The listing builds one solid part. Answer for the finished solid, in the listing's coordinates (mm). A direction names the side the tool comes from. Give positions to 0.01 mm unless a question says otherwise; leave off trailing zeros. Write each loop counter-clockwise with the first axis right and the second up, starting at its lowest first coordinate (ties: lowest second). Pieces come first, ordered by that corner, then holes. Notation, with made-up numbers: (64.5, 57) - (69.5, 57) arc R19 ccw to (69.5, 69) - close; hole circle Ø9 at (84, 55.5). An arc over 180 degrees is marked (long way). Return JSON: item names as keys, results as strings.
from build123d import *

# Parameters (mm, degrees)
F1_DEPTH = 10
F2_R     = 10
F3_T     = -1


with BuildPart() as f1:
    # F0 (on Top) → F1 (new body)
    with BuildSketch(Plane.XY):
        Polygon((35.284058, 50.538993), (-54.715942, 50.538993), (-54.715942, -39.461007), (-24.715942, -39.461007), (-24.715942, 20.538993), (5.284058, 20.538993), (5.284058, -39.461007), (35.284058, -39.461007), align=None)
    extrude(amount=F1_DEPTH)

    # F2
    f2_edges = [f1.edges().sort_by_distance(p)[0] for p in [
        (35.284058, 50.538993, 5),
        (35.284058, -39.461007, 5),
        (-24.715942, 20.538993, 5),
        (-24.715942, -39.461007, 5),
        (-54.715942, -39.461007, 5),
        (5.284058, -39.461007, 5),
        (5.284058, 20.538993, 5),
        (-54.715942, 50.538993, 5),
    ]]
    fillet(f2_edges, radius=F2_R)

    # F3
    f3_openings = [f1.faces().sort_by_distance(p)[0] for p in [
        (-9.715942, 49.2662, 10),
    ]]
    offset(amount=F3_T, openings=f3_openings)


solid = f1.part
Item 1: For faces 1 (the face through (20, -38.461, 5)), 2 (the face through (5.284, -9, 5)), 3 (the face through (-9, 50.539, 5)), determine the directions among +Z, -Z, +X, -X, +Y, -Y from which every point of the face is accessible in a straight line to the end or side of a thin tool.
Answer below:
{"face 1": "+Z", "face 2": "+Z, -Z, -Y", "face 3": "+Z, -Z, +X, -X, +Y"}
Item 2: A cutting plane is placed at C-C on y = 12. Determine the outline of the cut face in (x, z).
Answer below:
{"outline": "(-54.72, 0) - (-24.61, 0) - (-24.61, 10) - (-25.62, 10) - (-25.62, 1) - (-53.72, 1) - (-53.72, 10) - (-54.72, 10) - close; (5.18, 0) - (35.28, 0) - (35.28, 10) - (34.28, 10) - (34.28, 1) - (6.19, 1) - (6.19, 10) - (5.18, 10) - close"}
Item 3: Consider L1, parallel to X at y = 10, z = 1.5; L2, parallel to Y at x = 25, z = 3.25; L3, parallel to Y at x = -7, z = 9. Determine where each line is inside the solid, lowest interval first.
Answer below:
{"L1": "x = -54.72 to -53.72, -25.72 to -24.72, 5.28 to 6.28, 34.28 to 35.28", "L2": "y = -39.46 to -38.46, 49.54 to 50.54", "L3": "y = 20.54 to 21.54, 49.54 to 50.54"}
Item 4: A cutting plane is placed at D-D on x = 12.5. Determine the outline of the cut face in (y, z).
Answer below:
{"outline": "(-39.07, 0) - (50.54, 0) - (50.54, 10) - (49.54, 10) - (49.54, 1) - (-38.02, 1) - (-38.02, 10) - (-39.07, 10) - close"}
Item 5: A cutting plane is placed at A-A on y = 25.5. Determine the outline of the cut face in (x, z).
Answer below:
{"outline": "(-54.72, 0) - (35.28, 0) - (35.28, 10) - (34.28, 10) - (34.28, 1) - (-53.72, 1) - (-53.72, 10) - (-54.72, 10) - close"}
